CAD build for the part. Positions are in the model's coordinates, mm. Face numbers are marked on the shaded views. A direction names the side the tool comes from. Coordinates: 2 decimals unless noted, no trailing zeros. Write each loop counter-clockwise with the first axis right and the second up, starting at its lowest first coordinate (ties: lowest second). Pieces come first, ordered by that corner, then holes. Notation, with made-up numbers: (60, -21) -> (73, -21) arc R22 ccw to (73, 4) -> close; hole circle Ø10 at (42, 43.25). An arc over 180 degrees is marked (long way). Answer as CSV lines item,"result".
```python
from build123d import *

# Parameters (mm, degrees)
BOSS_EXTRUDE1_DEPTH            = 77
SKETCH3_W                      = 37.54
SKETCH3_H                      = 17.27
BOSS_EXTRUDE2_DEPTH            = 1.77
SKETCH4_W                      = 37.54
SKETCH4_H                      = 17.27
BOSS_EXTRUDE3_DEPTH            = 1.77
SKETCH5_W                      = 4
SKETCH5_H                      = 16
CUT_EXTRUDE2_DEPTH             = 1.77
SKETCH6_W                      = 9.78
SKETCH6_H                      = 11.05
SKETCH6_W_2                    = 7.24
SKETCH6_H_2                    = 7.24
BUTTON_WALLS_DEPTH             = 7.24
SKETCH7_W                      = 9.78
SKETCH7_H                      = 11.05
BUTTON_BOTTOM_DEPTH            = 1.27
SKETCH8_W                      = 7.24
SKETCH8_H                      = 1.77
BUTTON_CUTOUT_MIDDLE_DEPTH     = 7.24
SKETCH9_W                      = 4.45
SKETCH9_H                      = 1.27
SKETCH9_W_2                    = 3.37
SKETCH9_H_2                    = 4.39
BUTTON_CUTOUT_FRONT_BACK_DEPTH = 7.24
SKETCH10_W                     = 3.37
SKETCH10_H                     = 4.39
BUTTON_CUTOUT_BOTTOM_DEPTH     = 1.27
BUTTON_CHAMFER1_SIZE           = 5
SKETCH12_W                     = 35
SKETCH12_H                     = 1.77
SKETCH12_W_2                   = 1.77
SKETCH12_H_2                   = 10
SKETCH12_W_3                   = 7.5
SKETCH12_R                     = 0.9652
SKETCH12_H_3                   = 7
SUPPORT_PCB_BATTERY_DEPTH      = 7
SKETCH13_R                     = 1.25
SKETCH13_W                     = 8.8
SKETCH13_H                     = 4.8
CUTOUT_USB_3_LEDS_DEPTH        = 1.77
SKETCH16_W                     = 1.77
SKETCH16_H                     = 1.77
TAB_PCB_RETAINER_LEN_DEPTH     = 3
SKETCH17_W                     = 4
SKETCH17_H                     = 1.77
CUTOUT_BACK_MOT_WIRES_DEPTH    = 9
SKETCH18_R                     = 1.25
CUTOUT_CHG_DONE_LED_DEPTH      = 10
SKETCH19_W                     = 4.2
SKETCH19_H                     = 1.77
TAB_PCB_RETAINERS_WIDTH_DEPTH  = 10
CUTOUT_RETAINER_TAB_1_DEPTH    = 1.77
CUTOUT_RETAINER_TAB_2_DEPTH    = 1.77
SKETCH23_W                     = 8
SKETCH23_H                     = 8
SKETCH23_R                     = 0.9652
CASING_SCREW_POSTS_DEPTH       = 17.27


with BuildPart() as part:
    # Sketch2 → Boss-Extrude1 (new body)
    with BuildSketch(Plane.XY):
        Polygon((-30.215355805, 3.088014981), (-30.215355805, -12.911985019), (4.784644195, -12.911985019), (4.784644195, 3.088014981), (6.054644195, 3.088014981), (6.054644195, -14.181985019), (-31.485355805, -14.181985019), (-31.485355805, 3.088014981), align=None)
    extrude(amount=BOSS_EXTRUDE1_DEPTH)

    # Sketch3 → Boss-Extrude2 (add)
    with BuildSketch(Plane.XY.offset(77)):
        with Locations((-12.715355805, -5.546985019)):
            Rectangle(SKETCH3_W, SKETCH3_H)
    extrude(amount=BOSS_EXTRUDE2_DEPTH)

    # Sketch4 → Boss-Extrude3 (add)
    with BuildSketch(Plane(origin=(0, 0, 0), x_dir=(-1, 0, 0), z_dir=(0, 0, -1))):
        with Locations((12.715355805, -5.546985019)):
            Rectangle(SKETCH4_W, SKETCH4_H)
    extrude(amount=BOSS_EXTRUDE3_DEPTH)

    # Sketch5 → Cut-Extrude2 (cut)
    with BuildSketch(Plane(origin=(0, 0, -1.77), x_dir=(-1, 0, 0), z_dir=(0, 0, -1))):
        with Locations((19.215355805, -4.911985019)):
            Rectangle(SKETCH5_W, SKETCH5_H)
    extrude(amount=-CUT_EXTRUDE2_DEPTH, mode=Mode.SUBTRACT)

    # Sketch6 → button_walls (add)
    with BuildSketch(Plane(origin=(0, 3.088014981, 0), x_dir=(1, 0, 0), z_dir=(0, 1, 0))):
        with Locations((-7.725355805, 1.135)):
            Rectangle(SKETCH6_W, SKETCH6_H)
        with Locations((-7.725355805, 1.77)):
            Rectangle(SKETCH6_W_2, SKETCH6_H_2, mode=Mode.SUBTRACT)
    extrude(amount=-BUTTON_WALLS_DEPTH)

    # Sketch7 → button_bottom (add)
    with BuildSketch(Plane.XZ.offset(4.151985019)):
        with Locations((-7.725355805, -1.135)):
            Rectangle(SKETCH7_W, SKETCH7_H)
    extrude(amount=BUTTON_BOTTOM_DEPTH)

    # Sketch8 → button_cutout_middle (cut)
    with BuildSketch(Plane(origin=(0, 3.088014981, 0), x_dir=(1, 0, 0), z_dir=(0, 1, 0))):
        with Locations((-7.725355805, 0.885)):
            Rectangle(SKETCH8_W, SKETCH8_H)
    extrude(amount=-BUTTON_CUTOUT_MIDDLE_DEPTH, mode=Mode.SUBTRACT)

    # Sketch9 → button_cutout_front_back (cut)
    with BuildSketch(Plane(origin=(0, 3.088014981, 0), x_dir=(1, 0, 0), z_dir=(0, 1, 0))):
        with Locations((-7.720355805, 6.025)):
            Rectangle(SKETCH9_W, SKETCH9_H)
        with Locations((-10.930355805, -2.195)):
            Rectangle(SKETCH9_W_2, SKETCH9_H_2)
        with Locations((-4.520355805, -2.195)):
            Rectangle(SKETCH9_W_2, SKETCH9_H_2)
    extrude(amount=-BUTTON_CUTOUT_FRONT_BACK_DEPTH, mode=Mode.SUBTRACT)

    # Sketch10 → button_cutout_bottom (cut)
    with BuildSketch(Plane(origin=(0, -4.151985019, 0), x_dir=(1, 0, 0), z_dir=(0, 1, 0))):
        with Locations((-10.930355805, -2.195)):
            Rectangle(SKETCH10_W, SKETCH10_H)
        with Locations((-4.520355805, -2.195)):
            Rectangle(SKETCH10_W, SKETCH10_H)
    extrude(amount=-BUTTON_CUTOUT_BOTTOM_DEPTH, mode=Mode.SUBTRACT)

    # button_Chamfer1
    # the kernel refuses this chamfer: 5 mm, written as the material it adds along each edge
    with BuildSketch(Plane(origin=(-6.205355805, -5.421985019, 0), x_dir=(0, -0.9996219169112968, -0.027495876610586372), z_dir=(-1, 0, 0))) as button_chamfer1_piece_1_section:
        Polygon((BUTTON_CHAMFER1_SIZE * 0.999621916911, BUTTON_CHAMFER1_SIZE * 0.0274958766106), (-BUTTON_CHAMFER1_SIZE * 0.0274958766106, BUTTON_CHAMFER1_SIZE * 0.999621916911), (0, 0), align=None)
    button_chamfer1_piece_1 = extrude(amount=3.04, mode=Mode.PRIVATE)
    button_chamfer1_piece_1 = split(button_chamfer1_piece_1, bisect_by=Plane(origin=(-7.725355805, -7.110612501, 4.39), z_dir=(0, 0, -1)), keep=Keep.TOP, mode=Mode.PRIVATE)
    add(button_chamfer1_piece_1)

    # Sketch12 → support_pcb_battery (add)
    # profile 1 of 5: a face of its own
    with BuildSketch(Plane(origin=(0, -12.911985019, 0), x_dir=(1, 0, 0), z_dir=(0, 1, 0))):
        with Locations((-12.715355805, -76.115)):
            Rectangle(SKETCH12_W, SKETCH12_H)
    # profile 2 of 5: a face of its own
    with BuildSketch(Plane(origin=(0, -12.911985019, 0), x_dir=(1, 0, 0), z_dir=(0, 1, 0))):
        with Locations((-27.100355805, -60.23)):
            Rectangle(SKETCH12_W_2, SKETCH12_H_2)
    # profile 3 of 5: a face of its own
    with BuildSketch(Plane(origin=(0, -12.911985019, 0), x_dir=(1, 0, 0), z_dir=(0, 1, 0))):
        with Locations((1.034644195, -36.845)):
            Rectangle(SKETCH12_W_3, SKETCH12_H)
    # profile 4 of 5: a face of its own
    with BuildSketch(Plane(origin=(0, -12.911985019, 0), x_dir=(1, 0, 0), z_dir=(0, 1, 0))):
        with BuildLine():
            Line((-25.783918863, -37.73), (-19.764792747, -37.73))
            ThreePointArc((-19.764792747, -37.73), (-22.774355805, -30.7466), (-25.783918863, -37.73))
        make_face()
        with Locations(Location((-22.774355805, -34.8868, 0), (0, 0, 270))):
            Circle(SKETCH12_R, mode=Mode.SUBTRACT)
    # profile 5 of 5: a face of its own
    with BuildSketch(Plane(origin=(0, -12.911985019, 0), x_dir=(1, 0, 0), z_dir=(0, 1, 0))):
        with Locations((-12.100355805, -23.33)):
            Rectangle(SKETCH12_W_2, SKETCH12_H_3)
    extrude(amount=SUPPORT_PCB_BATTERY_DEPTH)

    # Sketch13 → cutout_usb_3_leds (cut)
    with BuildSketch(Plane(origin=(6.054644195, 0, 0), x_dir=(0, 0, -1), z_dir=(1, 0, 0))):
        with Locations((-51.3968, -3.411985019)):
            Circle(SKETCH13_R)
        with Locations((-47.5868, -3.411985019)):
            Circle(SKETCH13_R)
        with Locations((-24.2188, -3.411985019)):
            Circle(SKETCH13_R)
        with Locations((-34.8868, -3.411985019)):
            Rectangle(SKETCH13_W, SKETCH13_H)
    extrude(amount=-CUTOUT_USB_3_LEDS_DEPTH, mode=Mode.SUBTRACT)

    # Sketch16 → tab_pcb_retainer_len (add)
    with BuildSketch(Plane(origin=(0, -5.911985019, 0), x_dir=(1, 0, 0), z_dir=(0, 1, 0))):
        with Locations((-12.100355805, -20.715)):
            Rectangle(SKETCH16_W, SKETCH16_H)
    extrude(amount=TAB_PCB_RETAINER_LEN_DEPTH)

    # Sketch17 → cutout_back_mot_wires (cut)
    with BuildSketch(Plane(origin=(0, 3.088014981, 0), x_dir=(1, 0, 0), z_dir=(0, 1, 0))):
        with Locations((-20.361355805, -77.885)):
            Rectangle(SKETCH17_W, SKETCH17_H)
    extrude(amount=-CUTOUT_BACK_MOT_WIRES_DEPTH, mode=Mode.SUBTRACT)

    # Sketch18 → cutout_chg_done_led (cut)
    with BuildSketch(Plane(origin=(6.054644195, 0, 0), x_dir=(0, 0, -1), z_dir=(1, 0, 0))):
        with Locations((-28.5368, -3.411985019)):
            Circle(SKETCH18_R)
    extrude(amount=-CUTOUT_CHG_DONE_LED_DEPTH, mode=Mode.SUBTRACT)

    # Sketch19 → tab_pcb_retainers_width (add)
    with BuildSketch(Plane(origin=(0, -12.911985019, 0), x_dir=(1, 0, 0), z_dir=(0, 1, 0))):
        with Locations((-28.115355805, -68.615)):
            Rectangle(SKETCH19_W, SKETCH19_H)
        with Locations((-28.115355805, -46.115)):
            Rectangle(SKETCH19_W, SKETCH19_H)
        with Locations((-28.115355805, -28.115)):
            Rectangle(SKETCH19_W, SKETCH19_H)
    extrude(amount=TAB_PCB_RETAINERS_WIDTH_DEPTH)

    # Sketch20 → cutout_retainer_tab_1 (cut)
    with BuildSketch(Plane.XY.offset(69.5)):
        Polygon((-26.015355805, -12.911985019), (-26.015355805, -5.911985019), (-28.445355805, -10.120868481), (-28.445355805, -12.911985019), align=None)
    extrude(amount=-CUTOUT_RETAINER_TAB_1_DEPTH, mode=Mode.SUBTRACT)

    # Sketch21 → cutout_retainer_tab_2 (cut)
    with BuildSketch(Plane.XY.offset(47)):
        Polygon((-26.015355805, -5.911985019), (-28.445355805, -10.120868481), (-28.445355805, -12.911985019), (-26.015355805, -12.911985019), align=None)
    extrude(amount=-CUTOUT_RETAINER_TAB_2_DEPTH, mode=Mode.SUBTRACT)

    # Sketch23 → casing_screw_posts (add)
    # profile 1 of 3: a face of its own
    with BuildSketch(Plane.XZ.offset(14.181985019)):
        with Locations((2.054644195, 2.23)):
            Rectangle(SKETCH23_W, SKETCH23_H)
        with Locations(Location((2.054644195, 2.23, 0), (0, 0, 270))):
            Circle(SKETCH23_R, mode=Mode.SUBTRACT)
    # profile 2 of 3: a face of its own
    with BuildSketch(Plane.XZ.offset(14.181985019)):
        with Locations((-27.485355805, 2.23)):
            Rectangle(SKETCH23_W, SKETCH23_H)
        with Locations(Location((-27.485355805, 2.23, 0), (0, 0, 270))):
            Circle(SKETCH23_R, mode=Mode.SUBTRACT)
    # profile 3 of 3: a face of its own
    with BuildSketch(Plane.XZ.offset(14.181985019)):
        with BuildLine():
            Line((-16.715355805, 82.77), (-16.715355805, 78.77))
            Line((-16.715355805, 78.77), (-8.715355805, 78.77))
            Line((-8.715355805, 78.77), (-8.715355805, 82.77))
            ThreePointArc((-8.715355805, 82.77), (-12.715355805, 86.77), (-16.715355805, 82.77))
        make_face()
        with Locations(Location((-12.715355805, 82.77, 0), (0, 0, 270))):
            Circle(SKETCH23_R, mode=Mode.SUBTRACT)
    extrude(amount=-CASING_SCREW_POSTS_DEPTH)


solid = part.part
```
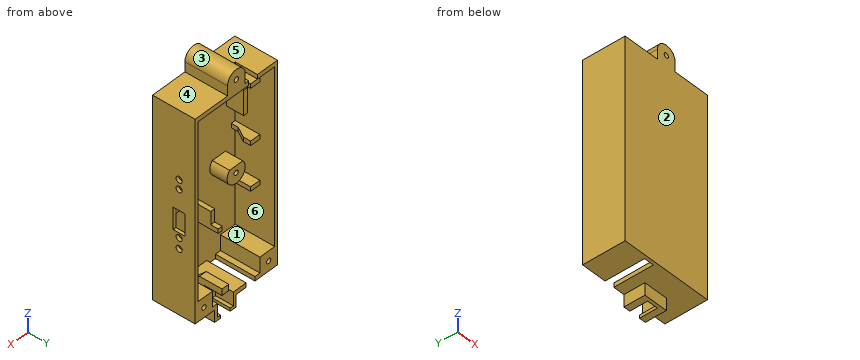
Item 1: Saw through at B-B on z = 9. Give the cut face in (x, y).
Answer below:
outline,"(-31.49, -14.18) -> (6.05, -14.18) -> (6.05, 3.09) -> (4.78, 3.09) -> (4.78, -12.91) -> (-30.22, -12.91) -> (-30.22, 3.09) -> (-31.49, 3.09) -> close"
Item 2: Two-plate mould, pull along Z, no slides. Class the marked faces 1, 2 and 3: pulls with the +Z half, pulls with the -Z half, needs draft (parallel to the pull), parting line crosses it, or undercut.
Answer below:
face 1,"undercut"
face 2,"needs draft"
face 3,"pulls with the +Z half"
Item 3: Wall check: line 1 (Z direction, x = 0, y = -12.25); line 2 (X direction, y = -0.25, z = 2.23); line 3 (Z direction, x = -5, y = -8.25). Give the ranges that are in metal, low to high. Write a range as from..to.
Answer below:
line 1,"z = -1.77..6.23, 35.96..37.73, 75.23..78.77"
line 2,"x = -31.49..-28.45, -26.52..-23.49, -9.25..-6.21, -1.95..1.09, 3.02..6.05"
line 3,"z = -1.77..0, 75.23..78.77"
Item 4: 3-axis set-ups, long thin cutter, end or side, ignore diameter. For the marked faces 4, 5 and 6: which of +Z, -Z, +X, -X, +Y, -Y reach the whole face in a straight line?
Answer below:
face 4,"+Z, +X, +Y, -Y"
face 5,"+Z, -X, +Y, -Y"
face 6,"+Y"
Item 5: Saw through at A-A on x = -7.5. Give the cut face in (y, z), and give its area (3 significant figures).
Answer below:
outline,"(-14.18, -1.77) -> (-5.42, -1.77) -> (-5.42, -6.66) -> (-4.15, -6.66) -> (-4.15, 1.85) -> (3.09, 1.85) -> (3.09, 4.39) -> (-6.03, 4.39) -> (-10.42, 0) -> (-12.91, 0) -> (-12.91, 75.23) -> (-5.91, 75.23) -> (-5.91, 77) -> (3.09, 77) -> (3.09, 78.77) -> (-14.18, 78.77) -> close"
area,"201 mm2"
Item 6: Saw through at D-D on z = 80. Give the cut face in (x, y), and give its area (3 significant figures).
Answer below:
outline,"(-16.72, -14.18) -> (-8.72, -14.18) -> (-8.72, 3.09) -> (-16.72, 3.09) -> close"
area,"138 mm2"
Item 7: Flat gauge pins, fed straight in: pin 1 (2 mm diameter, centred on x = -20.5, y = -9, fed in from -Z); pin 2 (2.5 mm diameter, centred on x = -22.5, y = -5, fed in from +Z); pin 3 (6 mm diameter, centred on x = -11, z = 14, fed in from +Y). Where does each tip first touch, or does it go through?
Answer below:
pin 1,"stops at z = -1.77"
pin 2,"stops at z = 78.77"
pin 3,"stops at y = -12.91"
Item 8: Saw through at C-C on x = -1. Give the cut face in (y, z).
Answer below:
outline,"(-14.18, -1.77) -> (3.09, -1.77) -> (3.09, 6.23) -> (-12.91, 6.23) -> (-12.91, 35.96) -> (-5.91, 35.96) -> (-5.91, 37.73) -> (-12.91, 37.73) -> (-12.91, 75.23) -> (-5.91, 75.23) -> (-5.91, 77) -> (3.09, 77) -> (3.09, 78.77) -> (-14.18, 78.77) -> close"
